Build history of the part. All positions in model axes, mm. Face numbers are marked on the shaded views. Give positions to 0.01 mm unless a question says otherwise; leave off trailing zeros. Order: outer loops, then holes, each group sorted by start corner. A loop starts at its lowest first (then second) coordinate and runs counter-clockwise, first axis right, second up. Notation, with made-up numbers: (55, 41.25) - (77, 41.25) arc R24 cw to (77, 59.25) - close; hole circle Ø10 at (34, 44.25). An arc over 180 degrees is marked (long way). One line per item, written item: value.
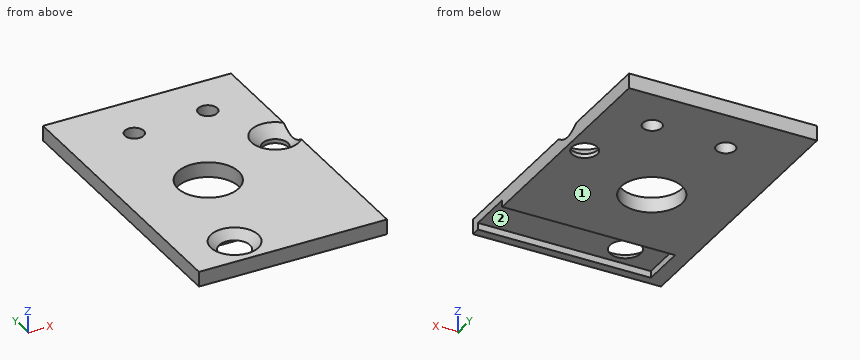
Autodesk Inventor part; units mm, degrees
ref_plane "YZ Plane" through (0, 0, 0) normal (1, 0, 0) x (0, 1, 0)
ref_plane "XZ Plane" through (0, 0, 0) normal (0, 1, 0) x (-1, 0, 0)
ref_plane "XY Plane" through (0, 0, 0) normal (0, 0, 1) x (1, 0, 0)
sketch "Szkic1" plane through (0, 0, 0) normal (0, 0, 1) x (1, 0, 0)
  line L0 (12.5, 18.6) -> (12.5, -19.4)
  line L1 (-12.5, 18.6) -> (12.5, 18.6)
  line L2 (12.5, -19.4) -> (-12.5, -19.4)
  line L3 (-12.5, -19.4) -> (-12.5, 18.6)
  line L4 (-12.5, 18.6) -> (12.5, 18.6)
  line L5 (12.5, 18.6) -> (12.5, -19.4)
extrude "Wyciągnięcie proste1" add sketch "Szkic1" along normal blind 2
sketch "Szkic2" plane through (0, 0, 2) normal (0, 0, 1) x (1, 0, 0)
  circle A0 centre (-3.9514, 12.0297) radius 1.25
  circle A1 centre (6.0405, 12.4305) radius 1.25
  circle A2 centre (-1.5, -1.5) radius 4.05
  circle A3 centre (10.2, 3.6) radius 1.2295
  point P0 (0, 0)
  point P1 (-5.5, -15.25)
extrude "Wyciągnięcie proste2" cut sketch "Szkic2" against normal through all contours A0 | A1 | A2
hole "Otwór1" at (10.2, 3.6, 2) at (-5.5, -15.25, 2) direction (0, 0, -1) diameter 3.4 depth 7 tip angle 118 countersink diameter 6.3 countersink angle 90
sketch "Szkic3" plane through (12.5, -18.6, 0) normal (1, 0, 0) x (0, 0, -1)
  line L0 (0, 0.4) -> (-0.9, 0.4)
  line L1 (-0.9, 0.4) -> (-0.9, 6.3)
  line L2 (-0.9, 6.3) -> (0, 6.3)
  line L3 (0, 6.3) -> (0, 0.4)
  point P0 (0, 18.6)
  dimension "d11" = 0.9
extrude "Wyciągnięcie proste3" cut sketch "Szkic3" against normal blind 23
properties part number "OslonaPrawejPrzekladni" material "Aluminium 6061"
(1) Pin check, flat tips, straight feed: P1, Ø1, axis at x = -0.5, y = -12.5, coming from the -Z side; P2, Ø1.8, axis at x = -4.5, y = -16.5, coming from the -Z side. Stop position of each tip, or through.
Completed:
P1: z = 0
P2: z = 0.9
(2) Pull direction Y, two halves, no side cores. Call the marked faces 1 and 2: +Y half, -Y half, draft (parallel to the pull), parting line (faces both ways), or undercut.
Completed:
face 1: draft
face 2: undercut
(3) Drill centre lines: line 1 (Y direction, x = 10.2, z = 0.3); line 2 (Y direction, x = -3, z = 1.05); line 3 (Y direction, x = 3.75, z = 0.75). Where is each one in solid material? Low to high.
Completed:
line 1: -19.4 to -18.2, -12.3 to 1.9, 5.3 to 18.6
line 2: -19.4 to -5.26, 2.26 to 11.22, 12.84 to 18.6
line 3: -19.4 to -18.2, -12.3 to 18.6
(4) Slice it at A-A, the plane y = -15.25. Give the cut face in (x, z), and give its area (3 significant figures).
Completed:
outline: (-12.5, 0) - (-10.5, 0) - (-10.5, 0.9) - (-7.55, 0.9) - (-8.65, 2) - (-12.5, 2) - close; (-3.45, 0.9) - (12.5, 0.9) - (12.5, 2) - (-2.35, 2) - close
area: 23.6 mm²
(5) Slice it at B-B, the plane x = -1.5. Give the cut face in (y, z).
Completed:
outline: (-19.4, 0) - (-18.2, 0) - (-18.2, 0.9) - (-12.3, 0.9) - (-12.3, 0) - (-5.55, 0) - (-5.55, 2) - (-19.4, 2) - close; (2.55, 0) - (18.6, 0) - (18.6, 2) - (2.55, 2) - close
(6) Slice it at D-D, the plane x = 10.2. Give the cut face in (y, z).
Completed:
outline: (-19.4, 0) - (-18.2, 0) - (-18.2, 0.9) - (-12.3, 0.9) - (-12.3, 0) - (1.9, 0) - (1.9, 0.55) - (0.45, 2) - (-19.4, 2) - close; (5.3, 0) - (18.6, 0) - (18.6, 2) - (6.75, 2) - (5.3, 0.55) - close
(7) Slice it at C-C, the plane y = -1.5. Give the cut face in (x, z), and give its area (3 significant figures).
Completed:
outline: (-12.5, 0) - (-5.55, 0) - (-5.55, 2) - (-12.5, 2) - close; (2.55, 0) - (12.5, 0) - (12.5, 2) - (2.55, 2) - close
area: 33.8 mm²
